Source: CAD feature listing. Evaluate the final solid. Frame: model axes, mm. A direction names the side the tool comes from. Round coordinates to 2 decimals unless told otherwise and drop trailing zeros. Write each loop counter-clockwise with the first axis right and the second up, starting at its lowest first coordinate (ties: lowest second). Pieces come first, ordered by that corner, then holes. Notation, with made-up numbers: M 65,20.5 L 107,20.5 A27 cw 107,45.5 Z; hole C 21,-21 d2. An arc over 180 degrees is marked long. Use a Markdown table: item, result.
```python
from build123d import *

# Parameters (mm, degrees)
F1_DEPTH = 2047.875
F3_DEPTH = 168.276
F5_DEPTH = 952.5
F7_DEPTH = 952.5


with BuildPart() as f1:
    # F0 (on Top) → F1 (new body)
    with BuildSketch(Plane.XY):
        Polygon((-19.05, 0), (0, 0), (0, 168.275), (-31.75, 168.275), (-31.75, 46.0375), (-19.05, 46.0375), align=None)
        Polygon((-933.45, 0), (-933.45, 46.0375), (-920.75, 46.0375), (-920.75, 168.275), (-952.5, 168.275), (-952.5, 0), align=None)
    extrude(amount=F1_DEPTH)

    # F2 (on Front) → F3 (cut, through all)
    with BuildSketch(Plane.XZ):
        Polygon((0, 2047.875), (-952.5, 2047.875), (-476.25, 1571.625), align=None)
    extrude(amount=-F3_DEPTH, mode=Mode.SUBTRACT)

    # F4 (on Right) → F5 (join, through all)
    with BuildSketch(Plane.YZ):
        Polygon((46.0375, 2016.125), (168.275, 2016.125), (168.275, 2047.875), (0, 2047.875), (0, 2028.825), (46.0375, 2028.825), align=None)
    extrude(amount=-F5_DEPTH)

    # F6 (on Right) → F7 (join, through all)
    with BuildSketch(Plane.YZ):
        Polygon((-17.4625, -12.7), (84.1375, -12.7), (185.7375, -12.7), (169.8625, 0), (84.1375, 0), (-1.5875, 0), align=None)
    extrude(amount=-F7_DEPTH)


solid = f1.part
```
Q1. Mould query, pull axis X, two halves, no side actions, for faces 1 (the flat face through (-470, 83, -12.7)), 2 (the flat face through (0, 83, 1032)), 3 (the flat face through (-952.5, 83, 1032)), 4 (the flat face through (-920.75, 106, 994)). Classes: +X half, -X half, draft (parallel to the pull), parting line (faces both ways), or undercut.
Results are:
| item | result |
|---|---|
| face 1 | draft |
| face 2 | +X half |
| face 3 | -X half |
| face 4 | undercut |
Q2. Section C-C on y = 120. Return loops of the section in (x, z) (3 decimals).
Results are:
| item | result |
|---|---|
| outline | M -952.5,-12.7 L 0,-12.7 L 0,2047.875 L -952.5,2047.875 Z; hole M -920.75,0 L -31.75,0 L -31.75,2016.125 L -920.75,2016.125 Z |
Q3. Section B-B on x = -752. Return loops of the section in (y, z) (1 decimal).
Results are:
| item | result |
|---|---|
| outline | M -17.5,-12.7 L 185.7,-12.7 L 169.9,0 L -1.6,0 Z; M 0,2028.8 L 46,2028.8 L 46,2016.1 L 168.3,2016.1 L 168.3,2047.9 L 0,2047.9 Z |
Q4. Reachability of faces 5 (the flat face through (-937, 0, 1019)), 6 (the flat face through (-31.75, 108, 994)), 7 (the flat face through (-933.45, 23, 1000)) from +Z, -Z, +X, -X, +Y, -Y: full face, straight path, thin tool, end or side. Return the list, or none.
Results are:
| item | result |
|---|---|
| face 5 | +Z, +X, -X, -Y |
| face 6 | +Y, -Y |
| face 7 | -Y |
Q5. Line query: L1, parallel to X at y = 144, z = 1788.5; L2, parallel to Z at x = -741.5, y = 71 (3 decimals); L3, parallel to X at y = 0.5, z = 1593.5. Output: solid intervals per line, ascending.
Results are:
| item | result |
|---|---|
| L1 | -952.5 to -920.75, -31.75 to 0 |
| L2 | -12.7 to 0, 2016.125 to 2047.875 |
| L3 | -952.5 to -933.45, -19.05 to 0 |
